from build123d import *

# Parameters (mm, degrees)
BOSS_EXTRUDE1_START   = 600
SKETCH1_R             = 57.281017464
SKETCH1_R_2           = 38.771715285
BOSS_EXTRUDE1_DEPTH   = 293
SKETCH1_R_3           = 57.28102
SKETCH1_R_4           = 38.771715
BOSS_EXTRUDE1_2_DEPTH = 293
BOSS_EXTRUDE1_3_DEPTH = 293
BOSS_EXTRUDE1_4_DEPTH = 293
SKETCH2_W             = 415.282978995
SKETCH2_H             = 1690.728499163
BOSS_EXTRUDE2_DEPTH   = 34
SKETCH6_R             = 9.313662058
CUT_EXTRUDE3_DEPTH    = 126


with BuildPart() as part:
    # Sketch1 → Boss-Extrude1 (new body)
    with BuildSketch(Plane.XY.offset(427.014108562).offset(BOSS_EXTRUDE1_START)):
        with Locations((1173.639225527, -317.201613393)):
            Circle(SKETCH1_R)
        with Locations((1173.639225527, -317.201613393)):
            Circle(SKETCH1_R_2, mode=Mode.SUBTRACT)
    extrude(amount=BOSS_EXTRUDE1_DEPTH)



with BuildPart() as body_2:
    # Sketch1 → Boss-Extrude1 2 (new body)
    with BuildSketch(Plane.XY.offset(427.014108562).offset(BOSS_EXTRUDE1_START)):
        with Locations((491.765116758, -317.201613393)):
            Circle(SKETCH1_R_3)
        with Locations((491.765116758, -317.201613393)):
            Circle(SKETCH1_R_4, mode=Mode.SUBTRACT)
    extrude(amount=BOSS_EXTRUDE1_2_DEPTH)


with BuildPart() as body_3:
    # Sketch1 → Boss-Extrude1 3 (new body)
    with BuildSketch(Plane.XY.offset(427.014108562).offset(BOSS_EXTRUDE1_START)):
        with Locations((491.765116758, -2112.860849235)):
            Circle(SKETCH1_R_3)
        with Locations((491.765116758, -2112.860849235)):
            Circle(SKETCH1_R_4, mode=Mode.SUBTRACT)
    extrude(amount=BOSS_EXTRUDE1_3_DEPTH)


with BuildPart() as body_4:
    # Sketch1 → Boss-Extrude1 4 (new body)
    with BuildSketch(Plane.XY.offset(427.014108562).offset(BOSS_EXTRUDE1_START)):
        with Locations((1173.639225527, -2112.860849235)):
            Circle(SKETCH1_R_3)
        with Locations((1173.639225527, -2112.860849235)):
            Circle(SKETCH1_R_4, mode=Mode.SUBTRACT)
    extrude(amount=BOSS_EXTRUDE1_4_DEPTH)


with BuildPart() as part_1:
    add(part.part)

    add(body_2.part)  # Boss-Extrude2 merges body 2

    add(body_3.part)  # Boss-Extrude2 merges body 3

    add(body_4.part)  # Boss-Extrude2 merges body 4
    # Sketch2 → Boss-Extrude2 (add)
    with BuildSketch(Plane(origin=(0, 0, 1027.014108562), x_dir=(-1, 0, 0), z_dir=(0, 0, -1))):
        Polygon((-1033.166693927, -2154.506262869), (-617.883714932, -2154.506262869), (-617.883714932, -2363.997444221), (-518.159541103, -2363.997444221), (-518.159541103, 172.765208514), (-617.883714932, 88.905828795), (-617.883714932, -284.095196719), (-1033.166693927, -284.095196719), (-1033.166693927, 91.617150216), (-1134.867510242, 172.765208514), (-1134.867510242, -2363.997444221), (-1033.166693927, -2363.997444221), align=None)
        with Locations((-825.52520443, -1232.946709341)):
            Rectangle(SKETCH2_W, SKETCH2_H, mode=Mode.SUBTRACT)
    extrude(amount=-BOSS_EXTRUDE2_DEPTH)

    # Sketch6 → Cut-Extrude3 (cut)
    with BuildSketch(Plane(origin=(0, -284.095196719, 0), x_dir=(1, 0, 0), z_dir=(0, 1, 0))):
        with Locations(Location((838.898443774, -1047.155157013, 0), (0, 0, 270))):
            Circle(SKETCH6_R)
    extrude(amount=-CUT_EXTRUDE3_DEPTH, mode=Mode.SUBTRACT)


solid = part_1.part
Design review of the part built by this model. Coordinates are the model's own, in mm. A direction names the side the tool comes from. Round coordinates to 2 decimals unless told otherwise and drop trailing zeros. Write each loop counter-clockwise with the first axis right and the second up, starting at its lowest first coordinate (ties: lowest second). Pieces come first, ordered by that corner, then holes. Notation, with made-up numbers: (17, 76) -> (31, 76) arc R11 cw to (31, 91) -> close; hole circle Ø4 at (47, -2.75). An arc over 180 degrees is marked (long way). One line per item, written item: value. Start each with the question number.
Q1. Insertion check: P1, Ø17, axis at x = 904, z = 1047.5, coming from the +Y side; P2, Ø17, axis at x = 794.5, z = 1046.5, coming from the -Y side; P3, Ø3.5, axis at x = 527, y = -2110.5, coming from the +Z side. Each pin has a flat end and moves straight along its axis. Give the tip position at first contact, or say it passes through.
Q2. Add section B-B (x = 725). Give the boundary of the cut face in (y, z), then the cut area to 3 significant figures.
Q3. Add section A-A (y = -1823). Give the boundary of the cut face in (x, z).
Q4. Add section C-C (z = 1163). Give the boundary of the cut face in (x, y).
Q5. To check wall thickness, follow probe 1 along Y at (x, z) = (1147, 1070); probe 2 along X at (y, z) = (-2140, 1103); probe 3 along X at (y, z) = (-2077, 1244.5). State the ranges of each line that lie inside material, in increasing order.
Q6. Add section D-D (x = 1157). Give the boundary of the cut face in (y, z).
Q7. The part is to be moulded in two halves that separate along X. For faces 4 (the face through (1211, -2125, 1320.014)), 5 (the face through (434.54, -314.68, 1171.46)), say which applies: pulls with the +X half, pulls with the -X half, needs draft (parallel to the pull), parting line crosses it, or undercut.
Q8. Tool access review of faces 1 (the face through (453.03, -2111.16, 1171.46)), 2 (the face through (529, -2125, 1320.014)), 3 (the face through (1083.305, 131.623, 1043.776)): name each direction out of +Z, -Z, +X, -X, +Y, -Y from which nothing blocks a thin tool from reaching the whole face with its end or side.
Response:
1. P1: stops at y = -284.1
1. P2: stops at y = -2154.51
1. P3: stops at z = 1061.01
2. outline: (-2154.51, 1027.01) -> (-2078.31, 1027.01) -> (-2078.31, 1061.01) -> (-2154.51, 1061.01) -> close; (-387.58, 1027.01) -> (-284.1, 1027.01) -> (-284.1, 1061.01) -> (-387.58, 1061.01) -> close
2. area: 6,110 mm^2
3. outline: (518.16, 1027.01) -> (617.88, 1027.01) -> (617.88, 1061.01) -> (518.16, 1061.01) -> close; (1033.17, 1027.01) -> (1134.87, 1027.01) -> (1134.87, 1061.01) -> (1033.17, 1061.01) -> close
4. outline: circle Ø114.56 at (491.77, -2112.86); circle Ø114.56 at (491.77, -317.2); circle Ø114.56 at (1173.64, -2112.86); circle Ø114.56 at (1173.64, -317.2); hole circle Ø77.54 at (491.77, -2112.86); hole circle Ø77.54 at (491.77, -317.2); hole circle Ø77.54 at (1173.64, -2112.86); hole circle Ø77.54 at (1173.64, -317.2)
5. probe 1: y = -2163.57 to -2141.03, -2084.69 to -2062.15, -367.91 to -345.37, -289.03 to -266.49
5. probe 2: x = 441.32 to 464.08, 519.45 to 542.21, 1123.2 to 1145.95, 1201.33 to 1224.08
5. probe 3: x = 447.1 to 477.03, 506.5 to 536.43, 1128.97 to 1158.9, 1188.38 to 1218.31
6. outline: (-2167.67, 1027.01) -> (-2147.88, 1027.01) -> (-2147.88, 1320.01) -> (-2167.67, 1320.01) -> close; (-2077.84, 1027.01) -> (-2058.05, 1027.01) -> (-2058.05, 1320.01) -> (-2077.84, 1320.01) -> close; (-372.01, 1027.01) -> (-352.22, 1027.01) -> (-352.22, 1320.01) -> (-372.01, 1320.01) -> close; (-282.18, 1027.01) -> (-262.39, 1027.01) -> (-262.39, 1320.01) -> (-282.18, 1320.01) -> close
7. face 4: needs draft
7. face 5: undercut
8. face 1: +Z
8. face 2: +Z, +X, -X, +Y, -Y
8. face 3: +Z, -Z, +Y
